Check sheet for the modelled part. Datum: model origin and axes. Units: mm. Round coordinates to 2 decimals unless told otherwise and drop trailing zeros. Order: outer loops, then holes, each group sorted by start corner. A loop starts at its lowest first (then second) coordinate and runs counter-clockwise, first axis right, second up.
```python
from build123d import *

# Parameters (mm, degrees)
F0_R     = 342.9
F0_R_2   = 254
F1_DEPTH = 226.939695


with BuildPart() as f1:
    # F0 (on Front) → F1 (new body)
    with BuildSketch(Plane.XZ):
        Polygon((364.206745, 1027.523371), (-729.422957, 0), (175.949275, -540.677786), (896.169722, 345.845073), (902.013715, 455.116268), align=None)
        Circle(F0_R, mode=Mode.SUBTRACT)
        with Locations((392.001907, 501.148325)):
            Circle(F0_R_2, mode=Mode.SUBTRACT)
    extrude(amount=F1_DEPTH)


solid = f1.part
```
Item 1: Sectioned sample at D-D (x = 793.5). Record the cut outline in (y, z), and give its area (3 significant figures).
Answer:
outline: (-226.94, 219.47) - (0, 219.47) - (0, 570.61) - (-226.94, 570.61) - close
area: 79,700 mm2
Item 2: Sectioned sample at A-A (x = 0). Record the cut outline in (y, z).
Answer:
outline: (-226.94, -435.6) - (0, -435.6) - (0, -342.9) - (-226.94, -342.9) - close; (-226.94, 342.9) - (0, 342.9) - (0, 685.33) - (-226.94, 685.33) - close
Item 3: Sectioned sample at B-B (z = -69). Record the cut outline in (x, y).
Answer:
outline: (-613.88, -226.94) - (-335.89, -226.94) - (-335.89, 0) - (-613.88, 0) - close; (335.89, -226.94) - (559.15, -226.94) - (559.15, 0) - (335.89, 0) - close
Item 4: Release check for a two-part mould opening along Z. For faces 1 (the flat face through (-283.074, -111.881, -266.554)), 2 (the flat face through (-174.953, -111.881, 520.954)), 3 (the cylindrical face through (184.341, -111.881, 289.135)), 4 (the cylindrical face through (138.248, -111.881, 512.316)) record: released by +Z, released by -Z, zero draft, split by the parting line, or undercut.
Answer:
face 1: released by -Z
face 2: released by +Z
face 3: undercut
face 4: undercut
Item 5: Sectioned sample at C-C (y = -143). Record the cut outline in (x, z).
Answer:
outline: (-729.42, 0) - (175.95, -540.68) - (896.17, 345.85) - (902.01, 455.12) - (364.21, 1027.52) - close; hole circle Ø685.8 at (0, 0); hole circle Ø508 at (392, 501.15)
Item 6: Go/stop test with flat-tipped pins: P1, Ø8, axis at x = -38.5, y = -137.5, coming from the -Z side; P2, Ø1, axis at x = -225, y = -130, coming from the +Z side; P3, Ø10, axis at x = 216.5, y = -130.5, coming from the -Z side. Record where each tip stops, or that it passes through.
Answer:
P1: stops at z = -415
P2: stops at z = 474.4
P3: stops at z = -496.92
Item 7: Scan lines: line 1 along X through (y, z) = (-82, 314); line 2 along X through (y, z) = (-38.5, -286); line 3 along Z through (x, y) = (236.5, -30). Record each from-to range of solid material in increasing order.
Answer:
line 1: x = -395.22 to -137.78, 137.78 to 220.27, 563.73 to 870.3
line 2: x = -250.51 to -189.17, 189.17 to 382.85
line 3: z = -466.15 to -248.29, 248.29 to 300.31, 701.98 to 907.54
